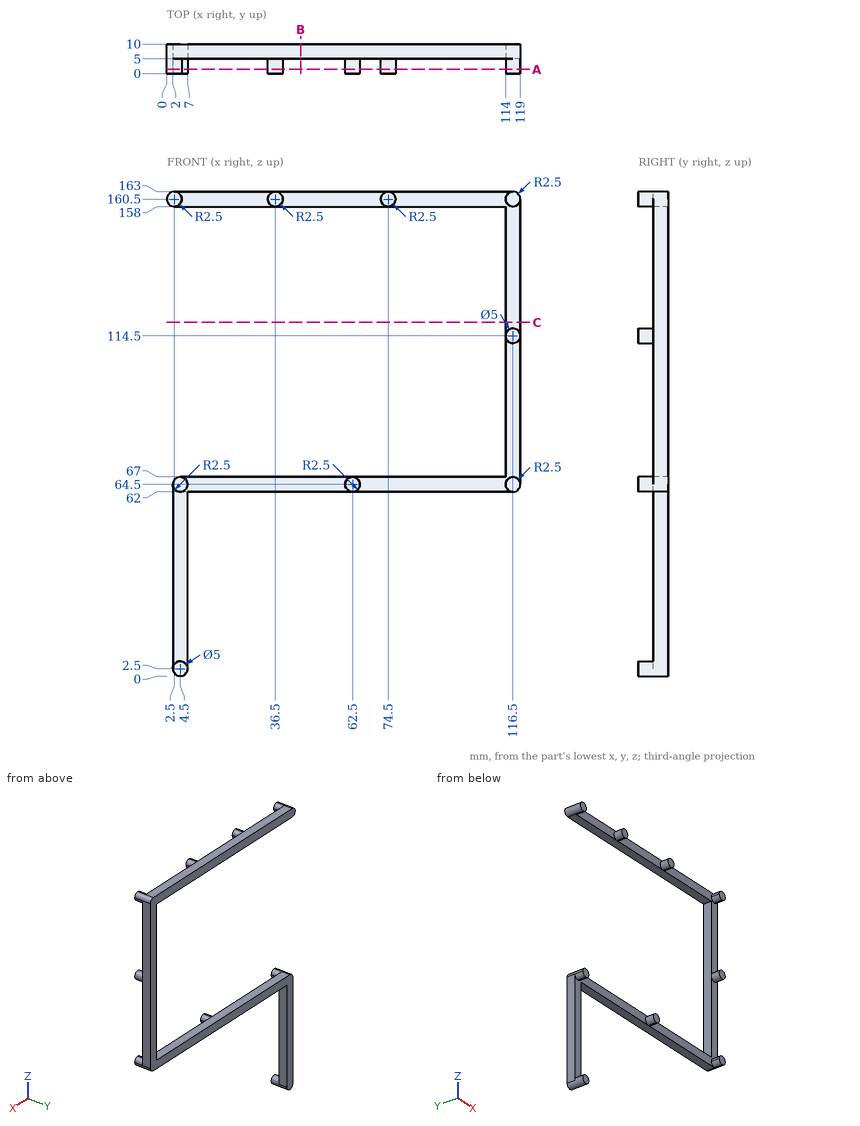
Job drawing, mm, ordinate dimensions from the low corner. One solid piece. Give positions to 0.01 mm unless a question says otherwise; leave off trailing zeros. Loops run counter-clockwise (first coordinate to the right, second up) from the corner with the lowest first, then second, coordinate; pieces in that order, holes last. Notation, with made-up numbers: (41.25, 79) - (62.25, 79) arc R17 ccw to (62.25, 92) - close; hole circle Ø2 at (78, 11.5). An arc over 180 degrees is marked (long way). Use one line per item in the form item = value.
(1) Cut at C-C (z = 119). Give the cut face in (x, y).
Determined:
outline = (114, 5) - (119, 5) - (119, 10) - (114, 10) - close
(2) Drill centre lines: L1, parallel to Z at x = 65.5, y = 5.5; L2, parallel to X at y = 6.75, z = 37.5; L3, parallel to X at y = 7.75, z = 99. Where is each one in solid material? Low to high.
Determined:
L1 = 62 to 67, 158 to 163
L2 = 2 to 7
L3 = 114 to 119
(3) Cut at B-B (x = 45). Give the cut face in (y, z).
Determined:
outline = (5, 62) - (10, 62) - (10, 67) - (5, 67) - close; (5, 158) - (10, 158) - (10, 163) - (5, 163) - close
(4) Cut at A-A (y = 1.5). Count the separate pieces of the cut face and the enclosed holes in it, then the cut area to 3 significant figures.
Determined:
separate_pieces = 9
enclosed_holes = 0
area = 177 mm^2
(5) Drop flat-ended pins along their axis: P1, Ø5, axis at y = 6.5, z = 123, coming from the -X side; P2, Ø2, axis at x = 50.5, y = 7.5, coming from the -Z side; P3, Ø4, axis at x = 19, z = 159.5, coming from the -Y side; P4, Ø1.5, axis at x = 99, y = 3.5, coming from the +Z side. Give the stop position or say it passes through.
Determined:
P1 = 114
P2 = 62
P3 = 5
P4 = through
